Autodesk Inventor part; units mm, degrees
ref_plane "Work Plane1" through (0, 1.2065, 3.1382) normal (0, 1, 0) x (0.866, 0, -0.5)
ref_plane "YZ Plane" through (0, 0, 0) normal (1, 0, 0) x (0, 1, 0)
ref_plane "XZ Plane" through (0, 0, 0) normal (0, 1, 0) x (-1, 0, 0)
sketch "Sketch1" plane through (0, 0, 0) normal (0, 1, 0) x (-1, 0, 0)
  line L0 (-2.7178, 1.5691) -> (0, 3.1382)
  line L1 (0, 3.1382) -> (2.7178, 1.5691)
  line L2 (2.7178, 1.5691) -> (2.7178, -1.5691)
  line L3 (2.7178, -1.5691) -> (0, -3.1382)
  line L4 (0, -3.1382) -> (-2.7178, -1.5691)
  line L5 (-2.7178, -1.5691) -> (-2.7178, 1.5691)
  circle A0 centre (0, 0) radius 1.5
  dimension "d1" = 3
extrude "Extrusion1" add sketch "Sketch1" along normal blind 2.413
thread "Thread1"
sketch "Sketch3" plane through (0, 0, 0) normal (1, 0, 0) x (0, 1, 0)
  line L0 (0, 3.1382) -> (2.413, 3.1382)
  line L1 (0, 1.5691) -> (0, 3.1382)
  line L2 (0, 1.5691) -> (0, 2.7572)
  line L3 (0.381, 3.1382) -> (2.413, 3.1382)
  arc A0 (0.381, 3.1382) -> (0, 2.7572) centre (0.381, 2.7572) ccw
  line L4 (0, 2.7572) -> (-0.2163, 2.7572)
  line L5 (-0.2163, 2.7572) -> (-0.2163, 4.3172)
  line L6 (-0.2163, 4.3172) -> (0.381, 4.3172)
  line L7 (0.381, 4.3172) -> (0.381, 3.1382)
  line L8 (-0.7421, 0) -> (2.9389, 0)
  point P0 (0, 0)
  dimension "d8" = 0.381
ref_plane "Work Plane1" through (0, 1.2065, 3.1382) normal (0, 1, 0) x (0.866, 0, -0.5)
revolve "Revolution2" cut sketch "Sketch3" angle 360 about axis through (0, -10, 0) along (0, 1, 0)
mirror "Mirror1" about plane through (0, 1.2065, 3.1382) normal (0, 1, 0) of "Revolution2"
properties part number "M3 nut"
Model file for the job. Use its own axes, mm. Give positions to 0.01 mm unless a question says otherwise; leave off trailing zeros. Loops run counter-clockwise (first coordinate to the right, second up) from the corner with the lowest first, then second, coordinate; pieces in that order, holes last.
1) Saw through at A-A (z = 0). Write the cut outline in (x, y).
2) Wall check: line 1 (Z direction, x = 0.9, y = 0.8); line 2 (Z direction, x = 0.5, y = 2.15); line 3 (X direction, y = 2.15, z = 0.5). Give the ranges that are in metal, low to high.
3) Saw through at B-B (y = 1.3). Write the cut outline in (x, z).
4) Pull direction X, two halves, no side cores. Call faces 1 (the flat face through (1.38, 1.19, 2.34)), 2 (the flat face through (-1.38, 1.19, -2.34)), 3 (the cylindrical face through (1.5, 1.19, -0.07)): +X half, -X half, draft (parallel to the pull), parting line (faces both ways), or undercut.
Answer block:
1. outline: (-2.72, 0) - (-1.5, 0) - (-1.5, 2.41) - (-2.72, 2.41) - close; (1.5, 0) - (2.72, 0) - (2.72, 2.41) - (1.5, 2.41) - close
2. line 1: z = -2.62 to -1.2, 1.2 to 2.62
2. line 2: z = -2.85 to -1.41, 1.41 to 2.85
2. line 3: x = -2.72 to -1.41, 1.41 to 2.72
3. outline: (-2.72, -1.57) - (0, -3.14) - (2.72, -1.57) - (2.72, 1.57) - (0, 3.14) - (-2.72, 1.57) - close; hole circle Ø3 at (0, 0)
4. face 1: +X half
4. face 2: -X half
4. face 3: undercut
